```python
from build123d import *

# Parameters (mm, degrees)
SKETCH_1_R          = 1.5
EXTRUDE_2_DEPTH     = 2
SKETCH_1_5_W        = 20
SKETCH_1_5_H        = 2.5
EXTRUDE_3_DEPTH     = 9.5
SKETCH_2_R          = 1.5
CUT_EXTRUDE_1_DEPTH = 18.036725037
FILLET_1_R          = 3
FILLET_2_R          = 2


with BuildPart() as part:
    # Sketch 1 → Extrude 2 (new body)
    with BuildSketch(Plane(origin=(0, 0, 0), x_dir=(1, 0, 0), z_dir=(0, 1, 0))):
        with BuildLine():
            Line((-10, -3.23), (10, -3.23))
            ThreePointArc((10, -3.23), (0, 6.77), (-10, -3.23))
        make_face()
        with Locations(Location((0, 0, 0), (0, 0, 270))):
            Circle(SKETCH_1_R, mode=Mode.SUBTRACT)
    extrude(amount=EXTRUDE_2_DEPTH)

    # Sketch 1_5 → Extrude 3 (add)
    with BuildSketch(Plane(origin=(0, 0, 0), x_dir=(1, 0, 0), z_dir=(0, 1, 0))):
        with Locations((0, -4.48)):
            Rectangle(SKETCH_1_5_W, SKETCH_1_5_H)
    extrude(amount=EXTRUDE_3_DEPTH)

    # Sketch 2 → Cut-Extrude 1 (cut, through all)
    with BuildSketch(Plane(origin=(0, 0, 3.23), x_dir=(-1, 0, 0), z_dir=(0, 0, -1))):
        with Locations((5, 6)):
            Circle(SKETCH_2_R)
        with Locations((-5, 6)):
            Circle(SKETCH_2_R)
    extrude(amount=-CUT_EXTRUDE_1_DEPTH, mode=Mode.SUBTRACT)

    # Fillet 1
    fillet_1_edges = [part.edges().sort_by_distance(p)[0] for p in [
        (-10, 9.5, 4.48),
        (10, 9.5, 4.48),
    ]]
    fillet(fillet_1_edges, radius=FILLET_1_R)

    # Fillet 2
    fillet_2_edges = [part.edges().sort_by_distance(p)[0] for p in [
        (0, 0, 5.73),
    ]]
    fillet(fillet_2_edges, radius=FILLET_2_R)


solid = part.part
```
Can you work these out from the model? Positions are in its coordinate system, mm. A direction names the side the tool comes from. Give positions to 0.01 mm unless a question says otherwise; leave off trailing zeros. Write each loop counter-clockwise with the first axis right and the second up, starting at its lowest first coordinate (ties: lowest second). Pieces come first, ordered by that corner, then holes. Notation, with made-up numbers: (43.25, 3) -> (88.25, 3) arc R33 cw to (88.25, 36) -> close; hole circle Ø10 at (48, 62). An arc over 180 degrees is marked (long way). Write item = value, one per line.
(1) Suppose I cut it at C-C on z = 3.5. Write out the boundary of the cut face in (x, y), then the cut area to 3 significant figures.
Worked out:
outline = (-10, 0) -> (10, 0) -> (10, 6.5) arc R3 ccw to (7, 9.5) -> (-7, 9.5) arc R3 ccw to (-10, 6.5) -> close; hole circle Ø3 at (-5, 6); hole circle Ø3 at (5, 6)
area = 172 mm^2
(2) Suppose I cut it at D-D on z = 0. Write out the boundary of the cut face in (x, y), then the cut area to 3 significant figures.
Worked out:
outline = (-9.46, 0) -> (-1.5, 0) -> (-1.5, 2) -> (-9.46, 2) -> close; (1.5, 0) -> (9.46, 0) -> (9.46, 2) -> (1.5, 2) -> close
area = 31.9 mm^2
(3) I need wall thicknesses on probe 1 along X at (y, z) = (6.75, 3.75); probe 2 along Y at (x, z) = (-5.5, -4.75); probe 3 along Z at (x, y) = (3.5, 5.5). Which ranges of each line are inside material? Lowest first, please. Write a range as from..to.
Worked out:
probe_1 = -9.99..-6.3, -3.7..3.7, 6.3..9.99
probe_2 = 0..2
probe_3 = 3.23..5.73
(4) I'm going to push flat-ended pins straight in: P1, Ø4, axis at x = 3.5, z = -4.5, coming from the +Y side; P2, Ø3, axis at x = 8, y = 6.5, coming from the -Z side; P3, Ø1, axis at y = 1, z = 0, coming from the +X side. Where does each tip first touch, or does it pass through?
Worked out:
P1 = 2
P2 = 3.23
P3 = 9.62
(5) Suppose I cut it at A-A on x = 0. Write out the boundary of the cut face in (y, z), then the cut area to 3 significant figures.
Worked out:
outline = (0, -6.77) -> (2, -6.77) -> (2, -1.5) -> (0, -1.5) -> close; (0, 1.5) -> (2, 1.5) -> (2, 3.23) -> (9.5, 3.23) -> (9.5, 5.73) -> (2, 5.73) arc R2 ccw to (0, 3.73) -> close
area = 36.9 mm^2
(6) For faces 1 (the face through (0, 2, -2)), 2 (the face through (10, 3, 4)), which set-ups out of +Z, -Z, +X, -X, +Y, -Y let a thin tool reach every point of the face, with its end or its side?
Worked out:
face_1 = -Z, +X, -X, +Y
face_2 = +Z, -Z, +X, +Y, -Y
(7) Thinking about a two-plate mould opening in X: for faces 3 (the face through (0, 0, -2)), 4 (the face through (9.1, 8.64, 4.46)), 5 (the face through (-6.386, 5.425, 4.462)), 6 (the face through (0.45, 0.99, 1.43)), which applies, released by +X, released by -X, zero draft, split by the parting line, or undercut?
Worked out:
face_3 = zero draft
face_4 = released by +X
face_5 = undercut
face_6 = undercut
(8) Suppose I cut it at B-B on y = 6. Write out the boundary of the cut face in (x, z), then the cut area to 3 significant figures.
Worked out:
outline = (-10, 3.23) -> (-6.5, 3.23) -> (-6.5, 5.73) -> (-10, 5.73) -> close; (-3.5, 3.23) -> (3.5, 3.23) -> (3.5, 5.73) -> (-3.5, 5.73) -> close; (6.5, 3.23) -> (10, 3.23) -> (10, 5.73) -> (6.5, 5.73) -> close
area = 35.0 mm^2
